from build123d import *

# Parameters (mm, degrees)
CHAMFER1_SIZE = 2


with BuildPart() as part:
    # Sketch1 → Revolve1 (revolve)
    with BuildSketch(Plane.XY, mode=Mode.PRIVATE) as revolve1_sk:
        with BuildLine():
            Line((0, 0), (141, 0))
            Line((141, 0), (141, 16))
            Line((141, 16), (111, 16))
            Line((111, 16), (111, 24))
            ThreePointArc((111, 24), (106, 29), (101, 24))
            Line((101, 24), (101, 16))
            Line((101, 16), (71, 16))
            ThreePointArc((71, 16), (66, 11), (61, 16))
            Line((61, 16), (31, 16))
            ThreePointArc((31, 16), (26.757359313, 17.757359313), (25, 22))
            Line((25, 22), (25, 30))
            Line((25, 30), (0, 30))
            Line((0, 30), (0, 0))
        make_face()
    revolve(revolve1_sk.sketch.rotate(Axis((-31.320754717, 0, 0), (1, 0, 0)), 90), axis=Axis((-31.320754717, 0, 0), (1, 0, 0)))

    # Chamfer1
    chamfer1_edges = [part.edges().sort_by_distance(p)[0] for p in [
        (141, 0, -16),
        (25, 0, -30),
        (0, 0, -30),
    ]]
    chamfer(chamfer1_edges, length=CHAMFER1_SIZE)


solid = part.part
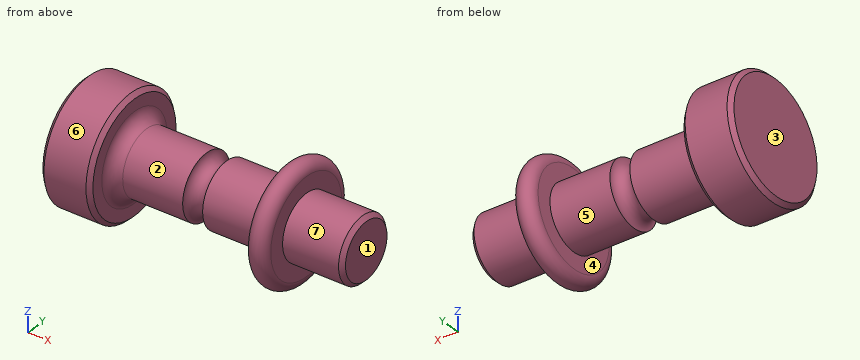
Geometry: final body of the model. Coordinates: model frame, mm. Face numbers are marked on the shaded views. A direction names the side the tool comes from. Give positions to 0.01 mm unless a question says otherwise; leave off trailing zeros. Loops run counter-clockwise (first coordinate to the right, second up) from the corner with the lowest first, then second, coordinate; pieces in that order, holes last. Notation, with made-up numbers: (29.25, -35.75) - (54.25, -35.75) arc R29 ccw to (54.25, -6.75) - close; hole circle Ø6 at (80, -3.75). An arc over 180 degrees is marked (long way). One line per question, with ' | ' between items. Start each with the question number.
(1) Pull-direction query (X, two-part tool) for the marked faces 1, 2, 3 and 4; classes: released by +X, released by -X, zero draft, split by the parting line, or undercut.
(2) Section query C-C on x = 118.5. Return loops of the section in (y, z), then the cut area to 3 significant figures.
(3) Contact query for flat-ended pins moving along their axis: pin 1 (8 mm diameter, centred on x = 75.5, y = -10, fed in from +Z); pin 2 (3 mm diameter, centred on x = 86.5, z = 7.5, fed in from +Y); pin 3 (2 mm diameter, centred on x = 118, z = 5.5, fed in from -Y); pin 4 (1.5 mm diameter, centred on y = -1.5, z = -9, fed in from -X). Output: stop coordinate, or through.
(4) Reachability of the marked faces 5, 6 and 7 from +Z, -Z, +X, -X, +Y, -Y: full face, straight path, thin tool, end or side. Return the list, or none.
(5) Ray query, line 1 (X direction, y = 8, z = 20); line 2 (X direction, y = -8, z = 10.5); line 3 (Y direction, x = 134, z = 0). Return the intervals inside material, ascending. Write a range as from..to.
(6) Section query A-A on y = 0. Return loops of the section in (x, z).
The answers:
1) face 1: released by +X | face 2: undercut | face 3: released by -X | face 4: undercut
2) outline: circle Ø32 at (0, 0) | area: 804 mm2
3) pin 1: z = 14.83 | pin 2: y = 14.83 | pin 3: y = -15.35 | pin 4: x = 0
4) face 5: none | face 6: +X, -X | face 7: +X
5) line 1: 0..25.02, 101..111 | line 2: 0..61.86, 70.14..141 | line 3: -16..16
6) outline: (0, -28) - (2, -30) - (23, -30) - (25, -28) - (25, -22) arc R6 cw to (31, -16) - (61, -16) arc R5 cw to (71, -16) - (101, -16) - (101, -24) arc R5 ccw to (111, -24) - (111, -16) - (139, -16) - (141, -14) - (141, 14) - (139, 16) - (111, 16) - (111, 24) arc R5 ccw to (101, 24) - (101, 16) - (71, 16) arc R5 cw to (61, 16) - (31, 16) arc R6 cw to (25, 22) - (25, 28) - (23, 30) - (2, 30) - (0, 28) - close
